Geometry check sheet. Reference: drawing and pictorial views, mm from the part's lowest x, y, z. Round coordinates to 2 decimals unless told otherwise and drop trailing zeros. Write each loop counter-clockwise with the first axis right and the second up, starting at its lowest first coordinate (ties: lowest second). Pieces come first, ordered by that corner, then holes.
Item 1: Depth check by flat-ended pin: pin 1 (2.5 mm diameter, centred on x = 55, z = 2, fed in from -Y); pin 2 (1.5 mm diameter, centred on x = 14.5, z = 3.5, fed in from +Y). Enter the tip coordinate at first touch or a pass-through.
Item 2: Material ranges on line 1 along X through (y, z) = (33.5, 2.45) (1 decimal); line 2 along Y through (x, z) = (17, 0.6), recorded low to high.
Item 3: Section check B-B, the plane z = 2.8. Record the cut outline in (x, y) (1 decimal).
Item 4: Section check A-A, the plane y = 42.5. Record the cut outline in (x, z) (1 decimal).
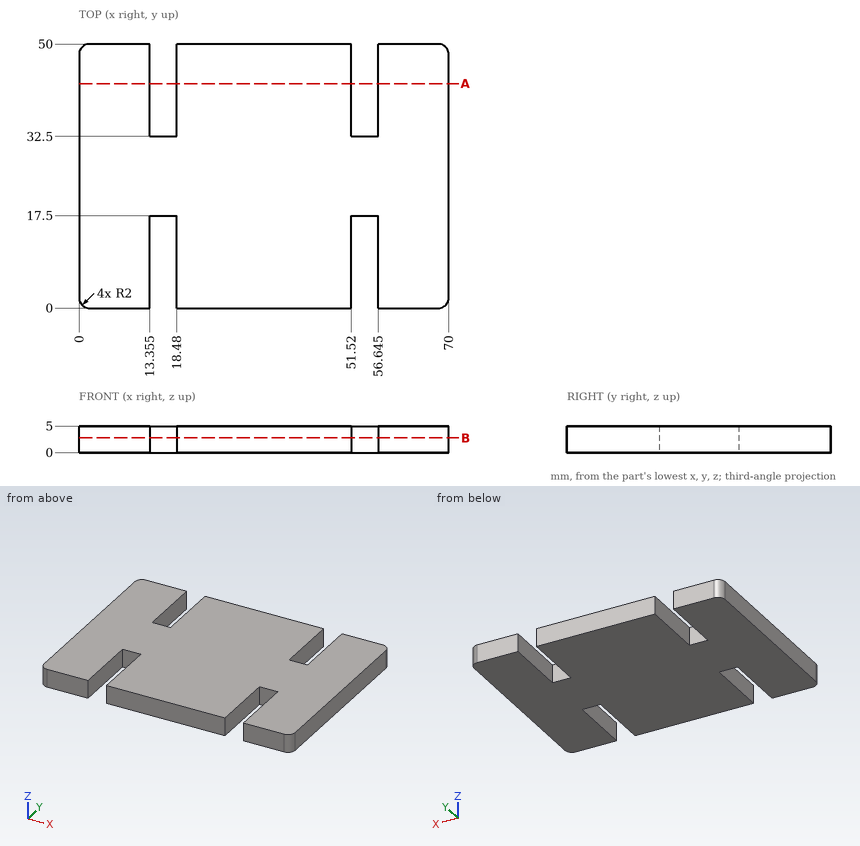
Values found:
1. pin 1: stops at y = 17.5
1. pin 2: stops at y = 32.5
2. line 1: x = 0 to 13.4, 18.5 to 51.5, 56.6 to 70
2. line 2: y = 17.5 to 32.5
3. outline: (0, 2) arc R2 ccw to (2, 0) - (13.4, 0) - (13.4, 17.5) - (18.5, 17.5) - (18.5, 0) - (51.5, 0) - (51.5, 17.5) - (56.6, 17.5) - (56.6, 0) - (68, 0) arc R2 ccw to (70, 2) - (70, 48) arc R2 ccw to (68, 50) - (56.6, 50) - (56.6, 32.5) - (51.5, 32.5) - (51.5, 50) - (18.5, 50) - (18.5, 32.5) - (13.4, 32.5) - (13.4, 50) - (2, 50) arc R2 ccw to (0, 48) - close
4. outline: (0, 0) - (13.4, 0) - (13.4, 5) - (0, 5) - close; (18.5, 0) - (51.5, 0) - (51.5, 5) - (18.5, 5) - close; (56.6, 0) - (70, 0) - (70, 5) - (56.6, 5) - close
